```python
from build123d import *

# Parameters (mm, degrees)
SKETCH1_W           = 409.575
SKETCH1_H           = 38.1
BOSS_EXTRUDE1_DEPTH = 6.35
CUT_EXTRUDE1_REACH  = 207.77
SKETCH2_W           = 3.175
SKETCH2_H           = 7.62
CUT_EXTRUDE2_REACH  = 207.77
SKETCH3_R           = 1.5


with BuildPart() as part:
    # Sketch1 → Boss-Extrude1 (new body)
    with BuildSketch(Plane(origin=(0, 0, 0), x_dir=(1, 0, 0), z_dir=(0, 1, 0))):
        Rectangle(SKETCH1_W, SKETCH1_H)
    extrude(amount=BOSS_EXTRUDE1_DEPTH)

    # Sketch2 → Cut-Extrude1 (cut, up to next)
    with BuildSketch(Plane(origin=(0, 6.35, 0), x_dir=(1, 0, 0), z_dir=(0, 1, 0)), mode=Mode.PRIVATE) as cut_extrude1_sk1:
        with Locations((-203.2, 7.62)):
            Rectangle(SKETCH2_W, SKETCH2_H)
    cut_extrude1_tool1 = extrude(cut_extrude1_sk1.sketch, amount=-CUT_EXTRUDE1_REACH, mode=Mode.PRIVATE) & part.part
    # Sketch2 → Cut-Extrude1 (cut, up to next)
    with BuildSketch(Plane(origin=(0, 6.35, 0), x_dir=(1, 0, 0), z_dir=(0, 1, 0)), mode=Mode.PRIVATE) as cut_extrude1_sk2:
        with Locations((-203.2, -7.62)):
            Rectangle(SKETCH2_W, SKETCH2_H)
    cut_extrude1_tool2 = extrude(cut_extrude1_sk2.sketch, amount=-CUT_EXTRUDE1_REACH, mode=Mode.PRIVATE) & part.part
    cut_extrude1_1 = cut_extrude1_tool1.solids().sort_by_distance((-203.2, 6.35, -7.62))[0]
    add(cut_extrude1_1, mode=Mode.SUBTRACT)
    cut_extrude1_2 = cut_extrude1_tool2.solids().sort_by_distance((-203.2, 6.35, 7.62))[0]
    add(cut_extrude1_2, mode=Mode.SUBTRACT)
    cut_extrude1 = cut_extrude1_1 + cut_extrude1_2  # Cut-Extrude1 as one shape, for the pattern or mirror that repeats it

    # Mirror1: Cut-Extrude1 across plane
    add(cut_extrude1.mirror(Plane(origin=(0, 0, 0), x_dir=(0, 0, 1), z_dir=(1, 0, 0))), mode=Mode.SUBTRACT)

    # Sketch3 → Cut-Extrude2 (cut, up to next)
    with BuildSketch(Plane(origin=(0, 6.35, 0), x_dir=(1, 0, 0), z_dir=(0, 1, 0)), mode=Mode.PRIVATE) as cut_extrude2_sk1:
        with Locations(Location((-138.1125, 6.717514421, 0), (0, 0, 270))):
            Circle(SKETCH3_R)
    cut_extrude2_tool1 = extrude(cut_extrude2_sk1.sketch, amount=-CUT_EXTRUDE2_REACH, mode=Mode.PRIVATE) & part.part
    # Sketch3 → Cut-Extrude2 (cut, up to next)
    with BuildSketch(Plane(origin=(0, 6.35, 0), x_dir=(1, 0, 0), z_dir=(0, 1, 0)), mode=Mode.PRIVATE) as cut_extrude2_sk2:
        with Locations(Location((-138.1125, -6.717514421, 0), (0, 0, 270))):
            Circle(SKETCH3_R)
    cut_extrude2_tool2 = extrude(cut_extrude2_sk2.sketch, amount=-CUT_EXTRUDE2_REACH, mode=Mode.PRIVATE) & part.part
    # Sketch3 → Cut-Extrude2 (cut, up to next)
    with BuildSketch(Plane(origin=(0, 6.35, 0), x_dir=(1, 0, 0), z_dir=(0, 1, 0)), mode=Mode.PRIVATE) as cut_extrude2_sk3:
        with Locations(Location((-124.677471157, 6.717514421, 0), (0, 0, 270))):
            Circle(SKETCH3_R)
    cut_extrude2_tool3 = extrude(cut_extrude2_sk3.sketch, amount=-CUT_EXTRUDE2_REACH, mode=Mode.PRIVATE) & part.part
    # Sketch3 → Cut-Extrude2 (cut, up to next)
    with BuildSketch(Plane(origin=(0, 6.35, 0), x_dir=(1, 0, 0), z_dir=(0, 1, 0)), mode=Mode.PRIVATE) as cut_extrude2_sk4:
        with Locations(Location((-124.677471157, -6.717514421, 0), (0, 0, 270))):
            Circle(SKETCH3_R)
    cut_extrude2_tool4 = extrude(cut_extrude2_sk4.sketch, amount=-CUT_EXTRUDE2_REACH, mode=Mode.PRIVATE) & part.part
    cut_extrude2_1 = cut_extrude2_tool1.solids().sort_by_distance((-138.1125, 6.35, -6.717514))[0]
    add(cut_extrude2_1, mode=Mode.SUBTRACT)
    cut_extrude2_2 = cut_extrude2_tool2.solids().sort_by_distance((-138.1125, 6.35, 6.717514))[0]
    add(cut_extrude2_2, mode=Mode.SUBTRACT)
    cut_extrude2_3 = cut_extrude2_tool3.solids().sort_by_distance((-124.677471, 6.35, -6.717514))[0]
    add(cut_extrude2_3, mode=Mode.SUBTRACT)
    cut_extrude2_4 = cut_extrude2_tool4.solids().sort_by_distance((-124.677471, 6.35, 6.717514))[0]
    add(cut_extrude2_4, mode=Mode.SUBTRACT)
    cut_extrude2 = cut_extrude2_1 + cut_extrude2_2 + cut_extrude2_3 + cut_extrude2_4  # Cut-Extrude2 as one shape, for the pattern or mirror that repeats it

    # Mirror2: Cut-Extrude2 across plane
    add(cut_extrude2.mirror(Plane(origin=(0, 0, 0), x_dir=(0, 0, 1), z_dir=(1, 0, 0))), mode=Mode.SUBTRACT)


solid = part.part
```
The model under review builds one solid part; all positions refer to its coordinate system, in mm. A direction names the side the tool comes from. Round coordinates to 2 decimals unless told otherwise and drop trailing zeros. Answer in a Markdown table with one row per item.
(1) Mouldability with a two-part tool opening along Z and no side actions: class faces 4 (the face through (-3, 3, -19.05)), 5 (the face through (201.612, 3, -8)), 6 (the face through (-204.788, 3, -15)) as released by +Z, released by -Z, zero draft, split by the parting line, or undercut.
Result set:
| item | result |
|---|---|
| face 4 | released by -Z |
| face 5 | undercut |
| face 6 | zero draft |
(2) Clearance check with flat-ended pins moving along their axes: P1, Ø1.5, axis at y = 3, z = 7.5, coming from the -X side; P2, Ø3, axis at y = 2, z = 6.5, coming from the +X side. State where each tip first meets the part, or that it passes through.
Result set:
| item | result |
|---|---|
| P1 | stops at x = -201.61 |
| P2 | stops at x = 201.61 |
(3) Machinability: for faces 1 (the face through (-3, 6.35, 0)), 2 (the face through (-201.612, 3, 8)), 3 (the face through (201.612, 3, 8)), which of the approach directions +Z, -Z, +X, -X, +Y, -Y give a long, thin tool a straight path to every point of the face, cutting with its end or side? Answer none if there is none.
Result set:
| item | result |
|---|---|
| face 1 | +Z, -Z, +X, -X, +Y |
| face 2 | -X, +Y, -Y |
| face 3 | +X, +Y, -Y |
(4) For line 1 (X direction, y = 4.5, z = -6); line 2 (X direction, y = 3, z = -8.5), list the stretches that pass through material, from the lowest coordinate up. Write a range as from..to.
Result set:
| item | result |
|---|---|
| line 1 | x = -201.61..-139.43, -136.8..-125.99, -123.36..123.36, 125.99..136.8, 139.43..201.61 |
| line 2 | x = -201.61..201.61 |
